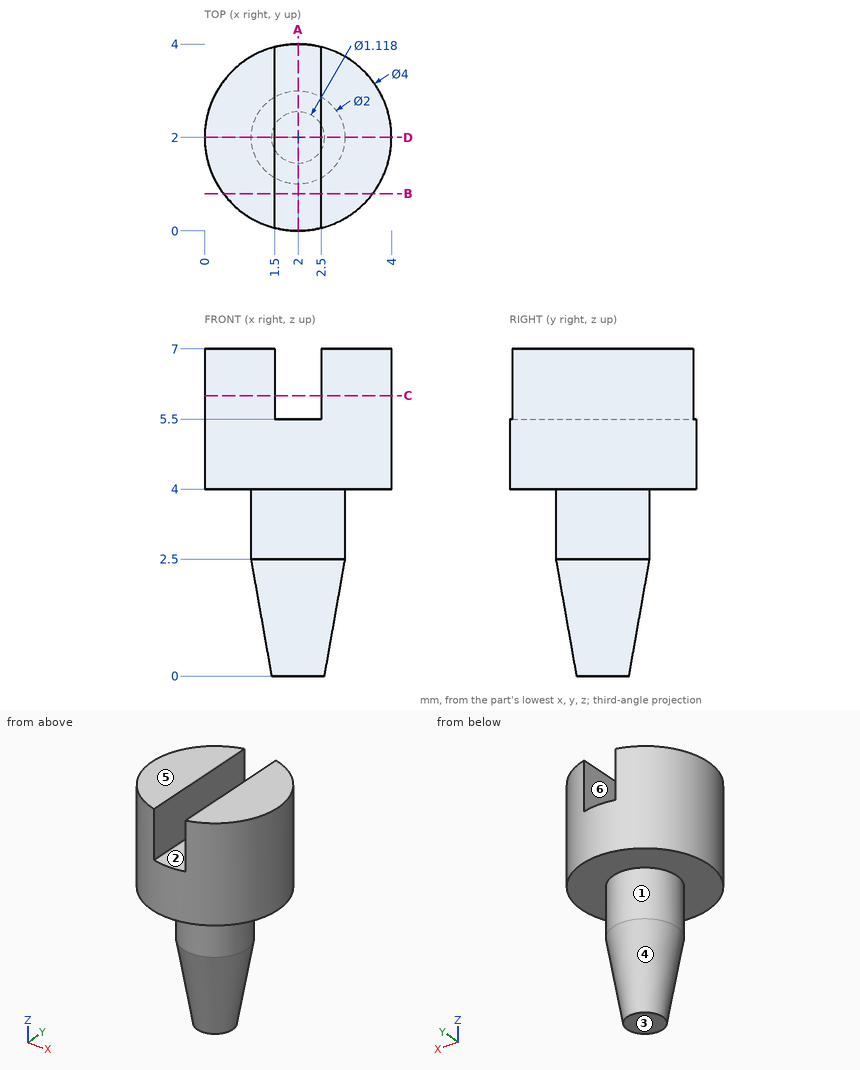
The drawing under review shows one solid part. Ordinate dimensions are in mm from its lowest x, y, z. A direction names the side the tool comes from. Coordinates: 2 decimals unless noted, no trailing zeros. Loops run counter-clockwise (first coordinate to the right, second up) from the corner with the lowest first, then second, coordinate; pieces in that order, holes last. Notation, with made-up numbers: (-19, 75) -> (32, 75) arc R9 ccw to (32, 90) -> close; hole circle Ø1 at (-14.5, 73). An arc over 180 degrees is marked (long way). Answer as a JSON object with one key per item and string values.
Q1. Clearance check with a flat-ended pin moving along its axis: pin 1 Ø0.5 at (x, y) = (2, 1.5) entering from +Z. State where the tip first meets the part, or that it passes through.
Answer block:
{"pin 1": "stops at z = 5.5"}
Q2. Take a section at B-B on y = 0.8. Give the boundary of the cut face in (x, z).
Answer block:
{"outline": "(0.4, 4) -> (3.6, 4) -> (3.6, 7) -> (2.5, 7) -> (2.5, 5.5) -> (1.5, 5.5) -> (1.5, 7) -> (0.4, 7) -> close"}
Q3. To check wall thickness, follow L1, parallel to Z at x = 0.45, y = 2.4; L2, parallel to Z at x = 1.6, y = 3.1; L3, parallel to X at y = 1.9, z = 6.25. State the ranges of each line that lie inside material, in increasing order.
Answer block:
{"L1": "z = 4 to 7", "L2": "z = 4 to 5.5", "L3": "x = 0 to 1.5, 2.5 to 4"}
Q4. The part is to be moulded in two halves that separate along X. For the marked faces 4, 5 and 6, say which applies: +X half, -X half, draft (parallel to the pull), parting line (faces both ways), or undercut.
Answer block:
{"face 4": "parting line", "face 5": "draft", "face 6": "undercut"}
Q5. Tool access review of the marked faces 1, 2 and 3: name each direction out of +Z, -Z, +X, -X, +Y, -Y from which nothing blocks a thin tool from reaching the whole face with its end or side.
Answer block:
{"face 1": "-Z", "face 2": "+Z, +Y, -Y", "face 3": "-Z, +X, -X, +Y, -Y"}
Q6. Take a section at A-A on x = 2. Give the boundary of the cut face in (y, z).
Answer block:
{"outline": "(0, 4) -> (1, 4) -> (1, 2.5) -> (1.44, 0) -> (2.56, 0) -> (3, 2.5) -> (3, 4) -> (4, 4) -> (4, 5.5) -> (0, 5.5) -> close"}
Q7. Take a section at C-C on z = 6. Give the boundary of the cut face in (x, y).
Answer block:
{"outline": "(1.5, 0.06) -> (1.5, 3.94) arc R2 ccw to start; (2.5, 0.06) arc R2 ccw to (2.5, 3.94) -> close"}
Q8. Take a section at D-D on y = 2. Give the boundary of the cut face in (x, z).
Answer block:
{"outline": "(0, 4) -> (1, 4) -> (1, 2.5) -> (1.44, 0) -> (2.56, 0) -> (3, 2.5) -> (3, 4) -> (4, 4) -> (4, 7) -> (2.5, 7) -> (2.5, 5.5) -> (1.5, 5.5) -> (1.5, 7) -> (0, 7) -> close"}
